Input: part model. Units: mm. Frame: model coordinates. Face numbers are marked on the shaded views. A direction names the side the tool comes from. Round coordinates to 2 decimals unless told otherwise and drop trailing zeros. Loops run counter-clockwise (first coordinate to the right, second up) from the corner with the lowest first, then second, coordinate; pieces in that order, holes last. Notation, with made-up numbers: (69.25, 50.5) -> (113.25, 50.5) arc R29 ccw to (113.25, 86.5) -> close; hole circle Ø3 at (-38.5, -30.75). An arc over 180 degrees is marked (long way). Answer as a JSON object with one key per item and string values.
```python
from build123d import *

# Parameters (mm, degrees)
SKETCH1_W           = 24
SKETCH1_H           = 60
BOSS_EXTRUDE1_DEPTH = 43
SKETCH2_W           = 24
SKETCH2_H           = 12.5
CUT_EXTRUDE1_DEPTH  = 11
SKETCH3_R           = 3.25
CUT_EXTRUDE2_DEPTH  = 33
SKETCH4_R           = 5
CUT_EXTRUDE3_DEPTH  = 2.5
SKETCH5_R           = 13
CUT_EXTRUDE4_DEPTH  = 25


with BuildPart() as part:
    # Sketch1 → Boss-Extrude1 (new body)
    with BuildSketch(Plane.XY):
        Rectangle(SKETCH1_W, SKETCH1_H)
    extrude(amount=BOSS_EXTRUDE1_DEPTH)

    # Sketch2 → Cut-Extrude1 (cut)
    with BuildSketch(Plane.XY.offset(43)):
        with Locations((0, -23.75)):
            Rectangle(SKETCH2_W, SKETCH2_H)
        with Locations((0, 23.75)):
            Rectangle(SKETCH2_W, SKETCH2_H)
    extrude(amount=-CUT_EXTRUDE1_DEPTH, mode=Mode.SUBTRACT)

    # Sketch3 → Cut-Extrude2 (cut, through all)
    with BuildSketch(Plane.XY.offset(32)):
        with Locations((-6.5, -23.75)):
            Circle(SKETCH3_R)
        with Locations((6.5, -23.75)):
            Circle(SKETCH3_R)
        with Locations((-6.5, 23.75)):
            Circle(SKETCH3_R)
        with Locations((6.5, 23.75)):
            Circle(SKETCH3_R)
    extrude(amount=-CUT_EXTRUDE2_DEPTH, mode=Mode.SUBTRACT)

    # Sketch4 → Cut-Extrude3 (cut)
    with BuildSketch(Plane.XY.offset(32)):
        with Locations((-6.5, 23.75)):
            Circle(SKETCH4_R)
        with Locations((6.5, 23.75)):
            Circle(SKETCH4_R)
        with Locations((-6.5, -23.75)):
            Circle(SKETCH4_R)
        with Locations((6.5, -23.75)):
            Circle(SKETCH4_R)
    extrude(amount=-CUT_EXTRUDE3_DEPTH, mode=Mode.SUBTRACT)

    # Sketch5 → Cut-Extrude4 (cut, through all)
    with BuildSketch(Plane(origin=(12, 0, 0), x_dir=(0, 0, -1), z_dir=(1, 0, 0))):
        with Locations((-25, 0)):
            Circle(SKETCH5_R)
    extrude(amount=-CUT_EXTRUDE4_DEPTH, mode=Mode.SUBTRACT)


solid = part.part
```
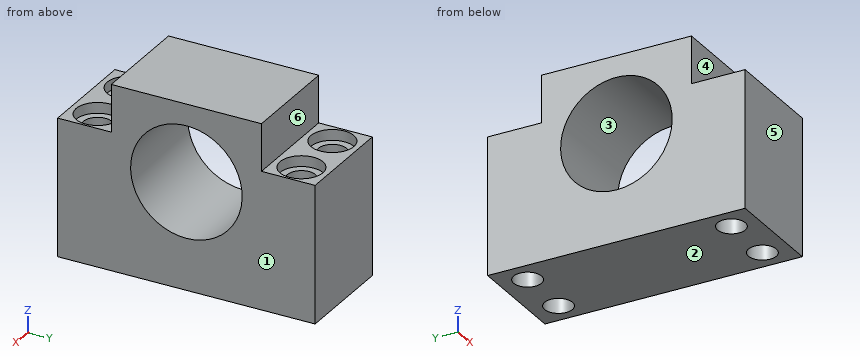
1) Contact query for flat-ended pins moving along their axis: P1, Ø8.5, axis at x = -6.5, y = 23.75, coming from the -Z side; P2, Ø5, axis at y = 1, z = 35, coming from the +X side; P3, Ø5.5, axis at x = -4, z = 35, coming from the -Y side; P4, Ø7.5, axis at x = 6.5, y = -23.75, coming from the +Z side. Output: stop coordinate, or through.
Output:
{"P1": "stops at z = 0", "P2": "passes through", "P3": "stops at y = -17.5", "P4": "stops at z = 29.5"}
2) Ray query, probe 1 along Y at (x, z) = (6.5, 31.05); probe 2 along X at (y, z) = (21, 26); probe 3 along Y at (x, z) = (6.5, 30.3). Return the intervals inside material, ascending.
Output:
{"probe 1": "y = -30 to -28.75, -18.75 to -11.51, 11.51 to 18.75, 28.75 to 30", "probe 2": "x = -12 to -8.23, -4.77 to 4.77, 8.23 to 12", "probe 3": "y = -30 to -28.75, -18.75 to -11.87, 11.87 to 18.75, 28.75 to 30"}
3) Draft query along Z for the marked faces 1, 2 and 3. Return one class per face: +Z half, -Z half, draft (parallel to the pull), parting line (faces both ways), or undercut.
Output:
{"face 1": "draft", "face 2": "-Z half", "face 3": "undercut"}
4) Reachability of the marked faces 4, 5 and 6 from +Z, -Z, +X, -X, +Y, -Y: full face, straight path, thin tool, end or side. Return the list, or none.
Output:
{"face 4": "+Z, +X, -X, -Y", "face 5": "+Z, -Z, +X, -X, -Y", "face 6": "+Z, +X, -X, +Y"}
5) Section B-B, the plane x = -6.5. Output: boundary loops of the cut face in (y, z), plus the area to 3 significant figures.
Output:
{"outline": "(-30, 0) -> (-27, 0) -> (-27, 29.5) -> (-28.75, 29.5) -> (-28.75, 32) -> (-30, 32) -> close; (-20.5, 0) -> (20.5, 0) -> (20.5, 29.5) -> (18.75, 29.5) -> (18.75, 32) -> (17.5, 32) -> (17.5, 43) -> (-17.5, 43) -> (-17.5, 32) -> (-18.75, 32) -> (-18.75, 29.5) -> (-20.5, 29.5) -> close; (27, 0) -> (30, 0) -> (30, 32) -> (28.75, 32) -> (28.75, 29.5) -> (27, 29.5) -> close; hole circle Ø26 at (0, 25)", "area": "1,340 mm^2"}
6) Section D-D, the plane x = 0.75. Output: boundary loops of the cut face in (y, z).
Output:
{"outline": "(-30, 0) -> (30, 0) -> (30, 32) -> (17.5, 32) -> (17.5, 43) -> (-17.5, 43) -> (-17.5, 32) -> (-30, 32) -> close; hole circle Ø26 at (0, 25)"}
7) Section C-C, the plane y = 0. Output: boundary loops of the cut face in (x, z).
Output:
{"outline": "(-12, 0) -> (12, 0) -> (12, 12) -> (-12, 12) -> close; (-12, 38) -> (12, 38) -> (12, 43) -> (-12, 43) -> close"}
8) Section A-A, the plane y = 23.75. Output: boundary loops of the cut face in (x, z).
Output:
{"outline": "(-12, 0) -> (-9.75, 0) -> (-9.75, 29.5) -> (-11.5, 29.5) -> (-11.5, 32) -> (-12, 32) -> close; (-3.25, 0) -> (3.25, 0) -> (3.25, 29.5) -> (1.5, 29.5) -> (1.5, 32) -> (-1.5, 32) -> (-1.5, 29.5) -> (-3.25, 29.5) -> close; (9.75, 0) -> (12, 0) -> (12, 32) -> (11.5, 32) -> (11.5, 29.5) -> (9.75, 29.5) -> close"}
